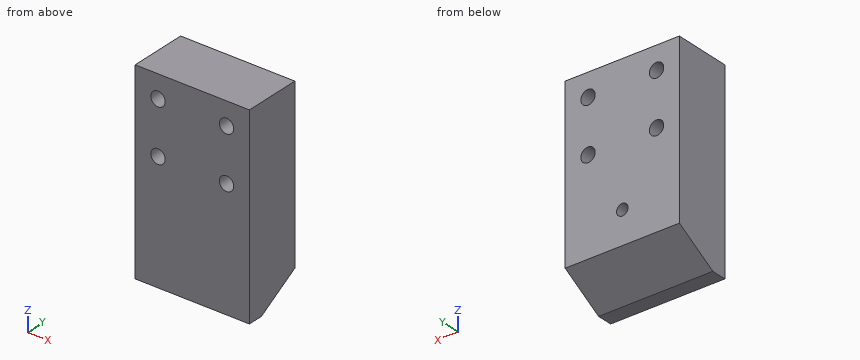
from build123d import *

# Parameters (mm, degrees)
PAD_DEPTH      = 17.5
SKETCH001_R    = 2.2
HOLE_DEPTH     = 17.632397
SKETCH002_R    = 1.75
HOLE001_DEPTH  = 13.948494
HOLE001_TIPS_R = 1.75


with BuildPart() as part:
    # Sketch → Pad (new body, symmetric)
    with BuildSketch(Plane.YZ):
        Polygon((30, 20), (30, 79.5), (47.631397, 79.5), (47.631397, 27.5), (34.641016, 20), align=None)
    extrude(amount=PAD_DEPTH, both=True)

    # Sketch001 (on Face3 of Pad) → Hole (cut, through all)
    with BuildSketch(Plane.ZX.offset(47.631397)):
        with Locations((72.5, 10.5)):
            Circle(SKETCH001_R)
        with Locations((56.5, 10.5)):
            Circle(SKETCH001_R)
        with Locations((56.5, -10.5)):
            Circle(SKETCH001_R)
        with Locations((72.5, -10.5)):
            Circle(SKETCH001_R)
    extrude(amount=-HOLE_DEPTH, mode=Mode.SUBTRACT)

    # Sketch002 (on Face11 of Hole) → Hole001 (cut)
    with BuildSketch(Plane.ZX.offset(47.631397)):
        with Locations((37.5, 0)):
            Circle(SKETCH002_R)
    extrude(amount=-HOLE001_DEPTH, mode=Mode.SUBTRACT)

    # Hole001 tips → Hole001 tip 1 section 0
    with BuildSketch(Plane.ZX.offset(33.682903), mode=Mode.PRIVATE) as hole001_tip_1_s0:
        with Locations((37.5, 0)):
            Circle(HOLE001_TIPS_R)
    loft([hole001_tip_1_s0.sketch, Vertex(0, 32.631397, 37.5)], mode=Mode.SUBTRACT)


solid = part.part
Design review of the part built by this model. Coordinates are the model's own, in mm. Coordinates: 2 decimals unless noted, no trailing zeros. Loops run counter-clockwise (first coordinate to the right, second up) from the corner with the lowest first, then second, coordinate; pieces in that order, holes last. Notation, with made-up numbers: M 60,6 L 107,6 A26 cw 107,31 Z; hole C 47.25,70.5 d10. An arc over 180 degrees is marked long. Use one line per item in the form item = value.
(1) For line 1 along X through (y, z) = (38.25, 56.5); line 2 along X through (y, z) = (46.5, 55.5); line 3 along X through (y, z) = (38.75, 37.5), list the stretches that pass through material, from the lowest coordinate up. Write a range as from..to.
Return value:
line_1 = -17.5..-12.7, -8.3..8.3, 12.7..17.5
line_2 = -17.5..-12.46, -8.54..8.54, 12.46..17.5
line_3 = -17.5..-1.75, 1.75..17.5
(2) Consider section D-D (x = 15). Write out the cut boundary in (y, z), and give its area (3 significant figures).
Return value:
outline = M 30,20 L 34.64,20 L 47.63,27.5 L 47.63,79.5 L 30,79.5 Z
area = 1,000 mm2
(3) Consider section A-A (z = 56.5). Write out the cut boundary in (x, y).
Return value:
outline = M -17.5,30 L -12.7,30 L -12.7,47.63 L -17.5,47.63 Z; M -8.3,30 L 8.3,30 L 8.3,47.63 L -8.3,47.63 Z; M 12.7,30 L 17.5,30 L 17.5,47.63 L 12.7,47.63 Z
(4) Clearance check with flat-ended pins moving along their axes: P1, Ø7, axis at x = 10.5, z = 56.5, coming from the -Y side; P2, Ø1, axis at x = -3.5, y = 42, coming from the -Z side; P3, Ø3, axis at x = 0, z = 37.5, coming from the +Y side. State where each tip first meets the part, or that it passes through.
Return value:
P1 = 30
P2 = 23.96
P3 = 33.53
(5) Consider section C-C (y = 41). Write out the cut boundary in (x, z), and give its area (3 significant figures).
Return value:
outline = M -17.5,23.67 L 17.5,23.67 L 17.5,79.5 L -17.5,79.5 Z; hole C -10.5,56.5 d4.4; hole C -10.5,72.5 d4.4; hole C 0,37.5 d3.5; hole C 10.5,56.5 d4.4; hole C 10.5,72.5 d4.4
area = 1,880 mm2
(6) Consider section B-B (x = 10.5). Write out the cut boundary in (y, z).
Return value:
outline = M 30,20 L 34.64,20 L 47.63,27.5 L 47.63,54.3 L 30,54.3 Z; M 30,58.7 L 47.63,58.7 L 47.63,70.3 L 30,70.3 Z; M 30,74.7 L 47.63,74.7 L 47.63,79.5 L 30,79.5 Z
